Verification items for the finished model (mm, model axes). A direction names the side the tool comes from. Give positions to 0.01 mm unless a question says otherwise; leave off trailing zeros. Write each loop counter-clockwise with the first axis right and the second up, starting at its lowest first coordinate (ties: lowest second). Pieces come first, ordered by that corner, then holes. Notation, with made-up numbers: (-20.75, -33.75) -> (3.25, -33.75) arc R15 ccw to (3.25, -10.75) -> close; hole circle Ø2 at (31.25, 84.5). An arc over 180 degrees is marked (long way). Answer as CSV lines item,"result". Start each with the question number.
1) Sectioned sample at C-C on z = 21.8. Record the cut outline in (x, y), and give its area (3 significant figures).
2) Tool access check on faces 4 (the cylindrical face through (29.97, -1.32, 2.54)), 5 (the flat face through (-0.5, 17, 8)), 6 (the flat face through (0, 10, 16)). Record the directions out of +Z, -Z, +X, -X, +Y, -Y that give a thin tool (end or side, any length) a straight path to the whole face; none if there is none.
3) Gauge pin test, flat ends, axial feed: pin 1 Ø4 at (x, y) = (15, 23) entering from +Z; pin 2 Ø4 at (x, z) = (17.5, 42) entering from -Y; pin 3 Ø8 at (x, z) = (0, 21.8) entering from +Y; pin 4 Ø1 at (y, z) = (-19, 31) entering from +X. Record the tip position at first contact, or that the pin passes through.
4) Mould release check, pull along Y, two halves, no side actions. Record for faces 1 (the cylindrical face through (-2.153, 15.153, 16.468)), 2 (the cylindrical face through (-0.651, 17.098, 16.843)), 3 (the flat face through (2, 24, 17)): released by +Y, released by -Y, zero draft, split by the parting line, or undercut.
5) Material ranges on L1, parallel to Y at x = 0, z = 2.1; L2, parallel to Y at x = 0, z = 34; L3, parallel to Z at x = 1, y = 17, recorded low to high.
6) Sectioned sample at D-D on z = 37.5. Record the cut outline in (x, y).
7) Sectioned sample at A-A on y = 0. Record the cut outline in (x, z), and give its area (3 significant figures).
8) Sectioned sample at B-B on z = 11. Record the cut outline in (x, y), and give its area (3 significant figures).
```python
from build123d import *

# Parameters (mm, degrees)
SKETCH012_W     = 1
SKETCH012_H     = 14
PAD004_DEPTH    = 21
SKETCH013_R     = 5.75
PAD005_DEPTH    = 14
SKETCH014_R     = 5
POCKET006_DEPTH = 14


with BuildPart() as part:
    # Sketch011 → Revolution (revolve)
    with BuildSketch(Plane.XZ):
        Polygon((0, 0), (-30, 0), (-30, 5), (-17, 28.3), (-17, 48.3), (-16.2, 48.3), (-16.2, 28.3), (-29.2, 5), (-29.2, 0.8), (0, 0.8), align=None)
    revolve(axis=Axis((0, 0, 0), (0, 0, 1)))

    # Sketch012 (on Face9 of Revolution) → Pad004 (new body)
    with BuildSketch(Plane(origin=(0, 0, 0.8), x_dir=(-1, 0, 0), z_dir=(0, 0, 1))):
        with Locations((0, -17)):
            Rectangle(SKETCH012_W, SKETCH012_H)
    extrude(amount=PAD004_DEPTH)

    # Sketch013 (on Face8 of Pad004) → Pad005 (join)
    with BuildSketch(Plane(origin=(0, 24, 0), x_dir=(1, 0, 0), z_dir=(0, 1, 0))):
        with Locations((0, -21.8)):
            Circle(SKETCH013_R)
    extrude(amount=-PAD005_DEPTH)

    # Sketch014 (on Face15 of Pad005) → Pocket006 (cut)
    with BuildSketch(Plane(origin=(0, 24, 0), x_dir=(1, 0, 0), z_dir=(0, 1, 0))):
        with Locations((0, -21.8)):
            Circle(SKETCH014_R)
    extrude(amount=-POCKET006_DEPTH, mode=Mode.SUBTRACT)


solid = part.part
```
Ans:
1,outline,"(-5.75, 10) -> (-5, 10) -> (-5, 24) -> (-5.75, 24) -> (-5.75, 19.81) arc R20.63 ccw (long way) to (5.75, 19.81) -> (5.75, 24) -> (5, 24) -> (5, 10) -> (5.75, 10) -> (5.75, 18.97) arc R19.83 cw (long way) to (-5.75, 18.97) -> close"
1,area,"113 mm²"
2,face 4,"+Z, -Z"
2,face 5,"none"
2,face 6,"+Z"
3,pin 1,"stops at z = 13.14"
3,pin 2,"stops at y = -6.98"
3,pin 3,"stops at y = -17.59"
3,pin 4,"passes through"
4,face 1,"undercut"
4,face 2,"zero draft"
4,face 3,"released by +Y"
5,L1,"y = -30 to -29.2, 10 to 24, 29.2 to 30"
5,L2,"y = -17 to -16.2, 16.2 to 17"
5,L3,"z = 0 to 0.8, 16.14 to 16.9, 26.7 to 28.25"
6,outline,"circle Ø34 at (0, 0); hole circle Ø32.4 at (0, 0)"
7,outline,"(-30, 0) -> (30, 0) -> (30, 5) -> (17, 28.3) -> (17, 48.3) -> (16.2, 48.3) -> (16.2, 28.3) -> (29.2, 5) -> (29.2, 0.8) -> (-29.2, 0.8) -> (-29.2, 5) -> (-16.2, 28.3) -> (-16.2, 48.3) -> (-17, 48.3) -> (-17, 28.3) -> (-30, 5) -> close"
7,area,"124 mm²"
8,outline,"circle Ø53.3 at (0, 0); (-0.5, 10) -> (0.5, 10) -> (0.5, 24) -> (-0.5, 24) -> close; hole circle Ø51.7 at (0, 0)"
8,area,"146 mm²"
